```python
from build123d import *

# Parameters (mm, degrees)
SKETCH_R           = 2.3
PAD_DEPTH          = 7.5
SKETCH001_R        = 2.3
PAD001_DEPTH       = 7.5
POCKET_DEPTH       = 44.4982971986
POLARPATTERN_COUNT = 3
POLARPATTERN_ANGLE = 180
FILLET_R           = 1
SKETCH003_W        = 15
SKETCH003_H        = 15
POCKET001_DEPTH    = 0.2
PAD002_DEPTH       = 8


with BuildPart() as part:
    # Sketch → Pad (new body, symmetric)
    with BuildSketch(Plane.XZ):
        Circle(SKETCH_R)
    extrude(amount=PAD_DEPTH, both=True)

    # Sketch001 → Pad001 (join)
    with BuildSketch(Plane.YZ):
        Circle(SKETCH001_R)
    extrude(amount=PAD001_DEPTH)

    # Sketch002 → Pocket (cut, through all)
    with BuildSketch(Plane.XZ):
        with BuildLine():
            ThreePointArc((-0.9641814145, 1.1490666647), (-1.4918817266, -0.1558490097), (-0.7058823529, -1.3235294118))
            Line((-0.7058823529, -1.3235294118), (0, -1.7))
            Line((0, -1.7), (0.7058823529, -1.3235294118))
            ThreePointArc((0.7058823529, -1.3235294118), (1.4918817266, -0.1558490097), (0.9641814145, 1.1490666647))
            Line((0.3076046329, 1.7), (0.9641814145, 1.1490666647))
            Line((-0.3076046329, 1.7), (0.3076046329, 1.7))
            Line((-0.9641814145, 1.1490666647), (-0.3076046329, 1.7))
        make_face()
    pocket = extrude(amount=-POCKET_DEPTH, mode=Mode.SUBTRACT)

    # PolarPattern: Pocket ×3 about axis
    polarpattern_axis = Axis((0, 0, 0), (0, 0, -1))
    for i in range(1, POLARPATTERN_COUNT):
        add(pocket.rotate(polarpattern_axis, i * POLARPATTERN_ANGLE / (POLARPATTERN_COUNT - 1)), mode=Mode.SUBTRACT)

    # Fillet
    fillet_edges = [part.edges().sort_by_distance(p)[0] for p in [
        (1.485912, -1.485912, 1.755581),
        (1.485912, 1.485912, 1.755581),
    ]]
    fillet(fillet_edges, radius=FILLET_R)

    # Sketch003 → Pocket001 (cut)
    with BuildSketch(Plane(origin=(0, 0, -2.3), x_dir=(-1, 0, 0), z_dir=(0, 0, -1))):
        Rectangle(SKETCH003_W, SKETCH003_H)
    extrude(amount=-POCKET001_DEPTH, mode=Mode.SUBTRACT)

    # Pocket001 Face10 → Pad002 (add)
    with BuildSketch(Plane(origin=(0, -7.5, 0.0372192642), x_dir=(-1, 0, 0), z_dir=(0, -1, 0))):
        with BuildLine():
            ThreePointArc((-2.3, 0.0372192642), (1.2514808729, -1.892494607), (0.938083152, 2.1372192642))
            Line((0.938083152, 2.1372192642), (-0.938083152, 2.1372192642))
            ThreePointArc((-0.938083152, 2.1372192642), (-1.9297138712, 1.2887001371), (-2.3, 0.0372192642))
        make_face()
        with BuildLine():
            ThreePointArc((-0.9641814145, -1.1118474005), (-1.4918817266, 0.1930682739), (-0.7058823529, 1.360748676))
            Line((-0.7058823529, 1.360748676), (0, 1.7372192642))
            Line((0, 1.7372192642), (0.7058823529, 1.360748676))
            ThreePointArc((0.7058823529, 1.360748676), (1.4918817266, 0.1930682739), (0.9641814145, -1.1118474005))
            Line((0.9641814145, -1.1118474005), (0.3076046329, -1.6627807358))
            Line((0.3076046329, -1.6627807358), (-0.3076046329, -1.6627807358))
            Line((-0.3076046329, -1.6627807358), (-0.9641814145, -1.1118474005))
        make_face(mode=Mode.SUBTRACT)
    extrude(amount=PAD002_DEPTH)


solid = part.part
```
Design review of the part built by this model. Coordinates are the model's own, in mm. A direction names the side the tool comes from. Coordinates: 2 decimals unless noted, no trailing zeros. Loops run counter-clockwise (first coordinate to the right, second up) from the corner with the lowest first, then second, coordinate; pieces in that order, holes last. Notation, with made-up numbers: (5.5, 50) - (25.5, 50) arc R14 ccw to (25.5, 62) - close; hole circle Ø8 at (-33.5, 76). An arc over 180 degrees is marked (long way). Use CSV: the item, a comma, the result in double quotes. Start each with the question number.
1) For pin 1 Ø1 at (y, z) = (-6.5, 1.5) entering from -X; pin 2 Ø1 at (y, z) = (3.5, 1.5) entering from +X; pin 3 Ø1 at (x, z) = (0.5, 0.5) entering from +Y, all flat-tipped, find the tip position at first contact; note any pin that passes through.
2) Consider section B-B on z = 0.7. Give the number of separate pieces and of enclosed holes in the cut face, then the cut area to 3 significant figures.
3) The part is to be moulded in two halves that separate along Z. For faces 1 (the flat face through (-2, -15.5, 0)), 2 (the cylindrical face through (4.055, 1.494, -0.135)), 3 (the flat face through (0, -3, -2.1)), say which applies: +Z half, -Z half, draft (parallel to the pull), parting line (faces both ways), or undercut.
4) Tool access review of faces 4 (the flat face through (2, 7.5, 0)), 5 (the cylindrical face through (4.06, -1.49, -0.18)), 6 (the cylindrical face through (1.49, 4.06, -0.18)): name each direction out of +Z, -Z, +X, -X, +Y, -Y from which nothing blocks a thin tool from reaching the whole face with its end or side.
5) Wall thickness on L1, parallel to Y at x = 5, z = 0; L2, parallel to Z at x = 0.5, y = -6.75 (3 decimals); L3, parallel to X at y = -10, z = 0.25: over which ranges is each line inside the solid? List them lowest first. Write a range as from..to.
6) Consider section A-A on y = -11.25. Write out the cut boundary in (x, z).
Geometry says:
1,pin 1,"x = -2.07"
1,pin 2,"x = 2.07"
1,pin 3,"through"
2,separate pieces,"3"
2,enclosed holes,"0"
2,area,"47.0 mm^2"
3,face 1,"draft"
3,face 2,"undercut"
3,face 3,"-Z half"
4,face 4,"+Z, -Z, +X, -X, +Y"
4,face 5,"+X"
4,face 6,"+Y, -Y"
5,L1,"-2.3..-1.5, 1.5..2.3"
5,L2,"-2.1..-1.433, 1.539..2.245"
5,L3,"-2.29..-1.48, 1.48..2.29"
6,outline,"(-0.94, -2.1) - (0.94, -2.1) arc R2.3 ccw (long way) to start; hole (-0.96, 1.15) arc R1.5 ccw to (-0.71, -1.32) - (0, -1.7) - (0.71, -1.32) arc R1.5 ccw to (0.96, 1.15) - (0.31, 1.7) - (-0.31, 1.7) - close"
